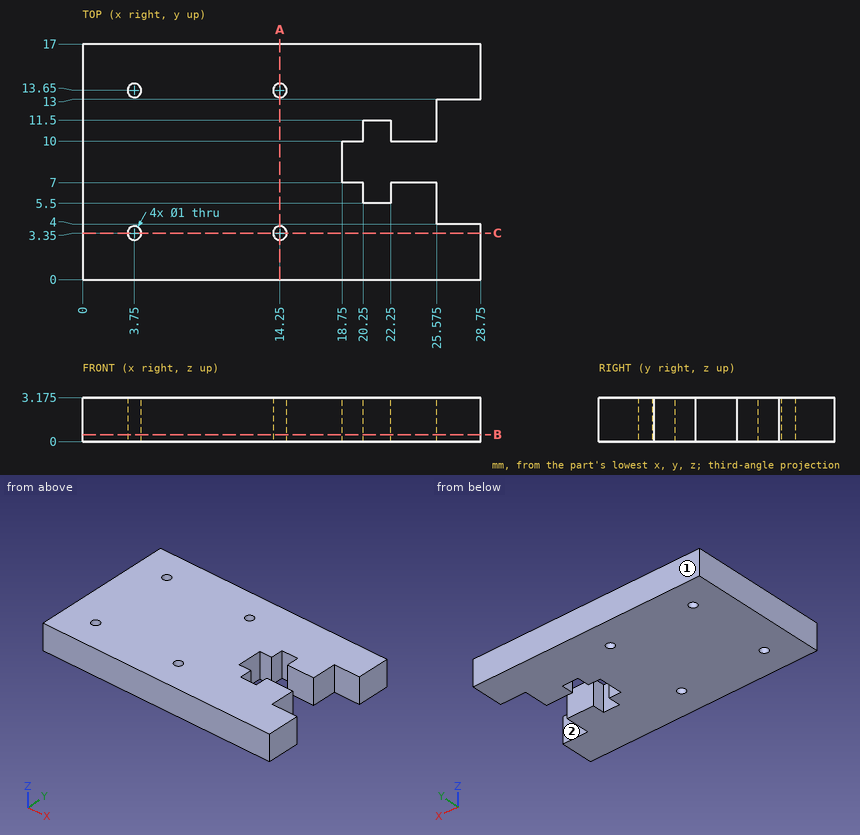
The drawing under review shows one solid part. Ordinate dimensions are in mm from its lowest x, y, z. A direction names the side the tool comes from. Coordinates: 2 decimals unless noted, no trailing zeros. Order: outer loops, then holes, each group sorted by start corner. A loop starts at its lowest first (then second) coordinate and runs counter-clockwise, first axis right, second up. Notation, with made-up numbers: (72.5, -4) - (81.5, -4) arc R22 cw to (81.5, 5) - close; hole circle Ø7 at (88, 84). An arc over 180 degrees is marked (long way). Put each result on its own line as item: value.
1) Take a section at B-B, the plane z = 0.5. Give the boundary of the cut face in (x, y) (3 decimals).
Response values:
outline: (0, 0) - (28.75, 0) - (28.75, 4) - (25.575, 4) - (25.575, 7) - (22.25, 7) - (22.25, 5.5) - (20.25, 5.5) - (20.25, 7) - (18.75, 7) - (18.75, 10) - (20.25, 10) - (20.25, 11.5) - (22.25, 11.5) - (22.25, 10) - (25.575, 10) - (25.575, 13) - (28.75, 13) - (28.75, 17) - (0, 17) - close; hole circle Ø1 at (3.75, 3.35); hole circle Ø1 at (3.75, 13.65); hole circle Ø1 at (14.25, 3.35); hole circle Ø1 at (14.25, 13.65)
2) Wall thickness on L1, parallel to X at y = 3.35, z = 1; L2, parallel to Y at x = 14.25, z = 0.8; L3, parallel to Y at x = 25.75, z = 1.3: over which ranges is each line inside the solid? List them lowest first. Write a range as from..to.
Response values:
L1: x = 0..3.25, 4.25..13.75, 14.75..28.75
L2: y = 0..2.85, 3.85..13.15, 14.15..17
L3: y = 0..4, 13..17
3) Take a section at A-A, the plane x = 14.25. Give the boundary of the cut face in (y, z) (3 decimals), and give its area (3 significant figures).
Response values:
outline: (0, 0) - (2.85, 0) - (2.85, 3.175) - (0, 3.175) - close; (3.85, 0) - (13.15, 0) - (13.15, 3.175) - (3.85, 3.175) - close; (14.15, 0) - (17, 0) - (17, 3.175) - (14.15, 3.175) - close
area: 47.6 mm²
4) Insertion check: P1, Ø1.6, axis at x = 21, z = 2.5, coming from the -Y side; P2, Ø1.6, axis at y = 6.5, z = 2, coming from the +X side (3 decimals). Each pin has a flat end and moves straight along its axis. Give the tip position at first contact, or say it passes through.
Response values:
P1: stops at y = 0
P2: stops at x = 25.575
5) Tool access review of the marked faces 1 and 2: name each direction out of +Z, -Z, +X, -X, +Y, -Y from which nothing blocks a thin tool from reaching the whole face with its end or side.
Response values:
face 1: +Z, -Z, +X, -X, +Y
face 2: +Z, -Z, +X
6) Take a section at C-C, the plane y = 3.35. Give the boundary of the cut face in (x, z) (3 decimals), and give its area (3 significant figures).
Response values:
outline: (0, 0) - (3.25, 0) - (3.25, 3.175) - (0, 3.175) - close; (4.25, 0) - (13.75, 0) - (13.75, 3.175) - (4.25, 3.175) - close; (14.75, 0) - (28.75, 0) - (28.75, 3.175) - (14.75, 3.175) - close
area: 84.9 mm²
